Geometry check sheet. Reference: the model listing, model coordinates, mm. Face numbers are marked on the shaded views. A direction names the side the tool comes from. Round coordinates to 2 decimals unless told otherwise and drop trailing zeros. Loops run counter-clockwise (first coordinate to the right, second up) from the corner with the lowest first, then second, coordinate; pieces in that order, holes last. Notation, with made-up numbers: M 22.25,13.5 L 50.25,13.5 A19 ccw 50.25,28.5 Z; hole C -35.75,44.25 d8. An arc over 180 degrees is marked long. Use one line per item in the form item = value. Start each with the question number.
1. Cross-section at A-A (z = 24.25). Record the boundary of the cut face in (x, y), then the cut area to 3 significant figures.
2. Material ranges on line 1 (Y direction, x = 25, z = 23.75); line 2 (Y direction, x = 45, z = 0.9); line 3 (Y direction, x = 25, z = 1.25), recorded low to high.
3. Cross-section at B-B (x = 6). State how many separate pieces and enclosed holes the cut face has, then the cut area to 3 significant figures.
4. Set-up check for the marked faces 1, 2, 3, 4 and 5: record each of +Z, -Z, +X, -X, +Y, -Y from which the full face is reachable in a straight line by a thin tool's end or side.
5. Go/stop test with flat-tipped pins: pin 1 (11.5 mm diameter, centred on x = 37.5, y = 9.5, fed in from +Z); pin 2 (3 mm diameter, centred on y = 19, z = 3, fed in from -X); pin 3 (2.5 mm diameter, centred on x = 25, z = 2, fed in from +Y); pin 4 (12 mm diameter, centred on x = 41.5, y = 38.5, fed in from -Z). Record where each tip stops, or that it passes through.
6. Cross-section at C-C (z = 7.5). Record the boundary of the cut face in (x, y), then the cut area to 3 significant figures.
7. Draft check along Y on the marked faces 6, 7 and 8. Enter one of: pulls with the +Y half, pulls with the -Y half, needs draft (parallel to the pull), parting line crosses it, or undercut.
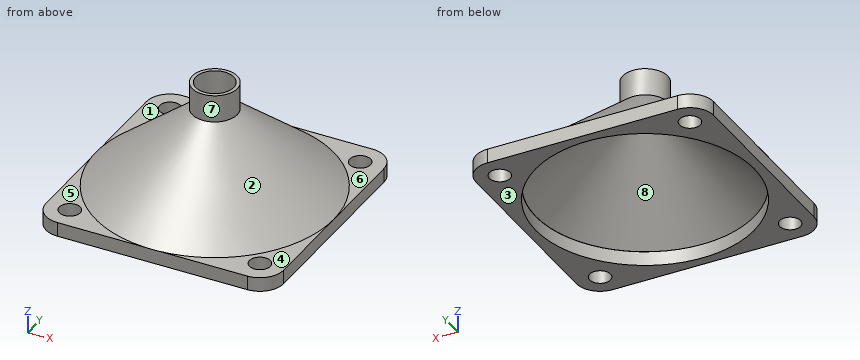
```python
from build123d import *

# Parameters (mm, degrees)
F0_W     = 50
F0_H     = 3
F1_DEPTH = 50
F2_R     = 23
F3_DEPTH = 25
F7_R     = 2.2
F8_DEPTH = 25
F9_R     = 5


with BuildPart() as f1:
    # F0 (on Front) → F1 (new body)
    with BuildSketch(Plane.XZ):
        with Locations((25, 1.5)):
            Rectangle(F0_W, F0_H)
    extrude(amount=-F1_DEPTH)

    # F2 (on face) → F3 (cut)
    with BuildSketch(Plane.XY.offset(3)):
        with Locations((25, 25)):
            Circle(F2_R)
    extrude(amount=-F3_DEPTH, mode=Mode.SUBTRACT)

    # F5 (on offset) → F6 (revolve)
    with BuildSketch(Plane.XZ.offset(-25)):
        Polygon((29.689003, 18.321594), (47.948567, 3), (50, 3), (29.689003, 20.04295), (29.689003, 25.803645), (28.947536, 25.803645), (28.947536, 18.321594), align=None)
    revolve(axis=Axis((24.948567, 25, 14.356404), (0, 0, 1)))

    # F7 (on face) → F8 (cut)
    with BuildSketch(Plane.XY.offset(3)):
        with Locations((45, 45)):
            Circle(F7_R)
        with Locations((45, 5)):
            Circle(F7_R)
        with Locations((5, 5)):
            Circle(F7_R)
        with Locations((5, 45)):
            Circle(F7_R)
    extrude(amount=-F8_DEPTH, mode=Mode.SUBTRACT)

    # F9
    f9_edges = [f1.edges().sort_by_distance(p)[0] for p in [
        (0, 0, 1.5),
        (50, 0, 1.5),
        (50, 50, 1.5),
        (0, 50, 1.5),
    ]]
    fillet(f9_edges, radius=F9_R)


solid = f1.part
```
Reported:
q1.outline = C 24.95,25 d9.48; hole C 24.95,25 d8
q1.area = 20.4 mm²
q2.line_1 = 20.26 to 21, 29 to 29.74
q2.line_2 = 0 to 2.8, 7.2 to 13.64, 36.36 to 42.8, 47.2 to 50
q2.line_3 = 0 to 2, 48 to 50
q3.separate_pieces = 3
q3.enclosed_holes = 0
q3.area = 99.5 mm²
q4.face_1 = +Z, -X, +Y
q4.face_2 = +Z
q4.face_3 = -Z, +X, -X, +Y, -Y
q4.face_4 = +Z, +X, -Y
q4.face_5 = +Z, -X, -Y
q5.pin_1 = 12.11
q5.pin_2 = 0
q5.pin_3 = 50.05
q5.pin_4 = 0
q6.outline = C 24.95,25 d39.38; hole C 24.95,25 d35.27
q6.area = 241 mm²
q7.face_6 = needs draft
q7.face_7 = parting line crosses it
q7.face_8 = undercut
